Autodesk Inventor part; units mm, degrees
ref_plane "YZ Plane" through (0, 0, 0) normal (1, 0, 0) x (0, 1, 0)
ref_plane "XZ Plane" through (0, 0, 0) normal (0, 1, 0) x (-1, 0, 0)
ref_plane "XY Plane" through (0, 0, 0) normal (0, 0, 1) x (1, 0, 0)
sketch "スケッチ1" plane through (0, 0, 0) normal (0, 1, 0) x (-1, 0, 0)
  arc A0 (0, -155) -> (25, -152.9706) centre (0, 0) ccw
  line L0 (25, -152.9706) -> (0, 0)
  line L1 (0, 0) -> (0, -144.6885)
  arc A1 (9.5, -144.6885) -> (23.3871, -143.1015) centre (0, 0) ccw
  line L2 (9.5, -144.6885) -> (9.5, -122.5)
  line L3 (9.5, -122.5) -> (0, -122.5)
  arc A2 (-25, -152.9706) -> (0, -155) centre (0, 0) ccw
  line L4 (-25, -152.9706) -> (0, 0)
  arc A3 (-23.3871, -143.1015) -> (-9.5, -144.6885) centre (0, 0) ccw
  line L5 (-9.5, -144.6885) -> (-9.5, -122.5)
  line L6 (-9.5, -122.5) -> (0, -122.5)
  line L7 (9.5, -144.6885) -> (0, -144.6885) construction
  line L8 (-9.5, -144.6885) -> (0, -144.6885) construction
  line L9 (-9.5, -180.2611) -> (-9.5, 6.4286)
  line L10 (9.5, -180.2611) -> (9.5, 6.4286)
  line L11 (0, -130) -> (-3.1667, -130)
  line L12 (-3.1667, -130) -> (-3.1667, -125)
  line L13 (-3.1667, -125) -> (0, -125)
  line L14 (0, -130) -> (3.1667, -130)
  line L15 (3.1667, -130) -> (3.1667, -125)
  line L16 (3.1667, -125) -> (0, -125)
  line L17 (0, -144.6885) -> (0, -145)
  line L18 (0, -145) -> (0, -155)
  point P0 (0, -125)
  point P1 (0, -150)
  dimension "d4" = 19
  dimension "d12" = 122.5
  dimension "d13" = 10
  dimension "d29" = 19
  dimension "d32" = 5
  dimension "d33" = 6.3333
  dimension "d34" = 2.5
  dimension "d36" = 50
  dimension "d38" = 150
extrude "押し出し1" add sketch "スケッチ1" along normal blind 1.6 contours L18 L17 L1 L14 L15 L16 L3 L2 L10 A0 | A2 L9 L5 L6 L1 L13 L12 L11 L17 L18 | L10 A1 L0 A0 | A2 L4 A3 L9
sketch "スケッチ2" plane through (0, 1.6, 0) normal (0, 1, 0) x (1, 0, 0)
  line L0 (9.5, 122.5) -> (9.5, 144.6885)
  arc A0 (23.3871, 143.1015) -> (9.5, 144.6885) centre (0, 0) ccw
  line L1 (23.3871, 143.1015) -> (25, 152.9706)
  arc A1 (25, 152.9706) -> (-25, 152.9706) centre (0, 0) ccw
  line L2 (-25, 152.9706) -> (-23.3871, 143.1015)
  arc A2 (-9.5, 144.6885) -> (-23.3871, 143.1015) centre (0, 0) ccw
  line L3 (-9.5, 144.6885) -> (-9.5, 122.5)
  line L4 (-9.5, 122.5) -> (9.5, 122.5)
  line L5 (-9.5, 122.5) -> (5.5, 122.5)
  line L6 (5.5, 122.5) -> (5.5, 132.5)
  line L7 (5.5, 132.5) -> (-9.5, 132.5)
  line L8 (-9.5, 132.5) -> (-9.5, 122.5)
  line L9 (-6.3333, 127.5) -> (-3.1667, 127.5) construction
  line L10 (-6.3333, 127.5) -> (-9.5, 127.5) construction
  line L11 (-3.1667, 125) -> (-3.1667, 130)
  point P0 (6.3333, 127.5)
  dimension "d19" = 10
  dimension "d20" = 15
hole "穴1" at (6.3333, 1.6, -127.5) at (-6.3333, 1.6, -127.5) direction (0, -1, 0) diameter 2.4 depth 1.6
fillet "フィレット1" radius 10 2 edges at (9.5, 0.8, -144.6885) (-9.5, 0.8, -144.6885)
fillet "フィレット2" radius 1.5 4 edges at (-3.1667, 0.8, -130) (3.1667, 0.8, -125) (3.1667, 0.8, -130) (-3.1667, 0.8, -125)
properties part number "sensor" material "エポキシ樹脂"
Read the model definition and answer for the solid it produces. Units are mm, in the model's axes. A direction names the side the tool comes from. Give positions to 0.01 mm unless a question says otherwise; leave off trailing zeros. Loops run counter-clockwise (first coordinate to the right, second up) from the corner with the lowest first, then second, coordinate; pieces in that order, holes last. Notation, with made-up numbers: M 84,-25 L 111,-25 A16 ccw 111,-11 Z; hole C 18.25,62 d11. An arc over 180 degrees is marked long. Write each question's results on one line, items separated by ' | '.
1. Section C-C on y = 0.5 is taken. Give the vertices of the cut face in (x, z).
Values:
outline: M -25,-152.97 A155 ccw 0,-155 A155 ccw 25,-152.97 L 23.39,-143.1 A145.02 cw 20.94,-143.48 A10 cw 9.5,-133.58 L 9.5,-122.5 L -9.5,-122.5 L -9.5,-133.58 A10 cw -20.94,-143.48 A144.98 cw -23.39,-143.1 Z; hole C -6.33,-127.5 d2.4; hole M -3.17,-128.5 A1.5 ccw -1.67,-130 L 1.67,-130 A1.5 ccw 3.17,-128.5 L 3.17,-126.5 A1.5 ccw 1.67,-125 L -1.67,-125 A1.5 ccw -3.17,-126.5 Z; hole C 6.33,-127.5 d2.4
2. A tool of negligible diameter and unlimited length cuts with its end or side. For faces 1 (the face through (9.5, 1, -128)), 2 (the face through (0, 0, -142)), 3 (the face through (22.15, 0.79, -143.3)), 4 (the face through (2.74, 0.81, -129.55)), 5 (the face through (0, 1.6, -142)), from which of +Z, -Z, +X, -X, +Y, -Y can it reach the whole face along a straight path? Write none if from no direction.
Values:
face 1: +Z, +X, +Y, -Y | face 2: +Z, -Z, +X, -X, -Y | face 3: +Z, +Y, -Y | face 4: +Y, -Y | face 5: +Z, -Z, +X, -X, +Y
3. Section B-B on x = 7 is taken. Give the vertices of the cut face in (y, z), plus the area to 3 significant figures.
Values:
outline: M 0,-154.84 L 1.6,-154.84 L 1.6,-128.5 L 0,-128.5 Z; M 0,-126.5 L 1.6,-126.5 L 1.6,-122.5 L 0,-122.5 Z | area: 48.6 mm^2
4. The mould has two halves that part along Z. Classify faces 6 (the face through (-12.87, 0.81, -141.07)), 7 (the face through (-12.716, 0.789, -154.477)), 8 (the face through (-3.167, 1, -128)): pulls with the +Z half, pulls with the -Z half, needs draft (parallel to the pull), parting line crosses it, or undercut.
Values:
face 6: pulls with the +Z half | face 7: pulls with the -Z half | face 8: undercut
5. Straight lines are drawn through the part: line 1 (X direction, y = 0.8, z = -127.5); line 2 (Z direction, x = 0, y = 0.25); line 3 (X direction, y = 1.1, z = -131). For each, find the intervals that lie inside material, in ascending order. Write a range as [from, to].
Values:
line 1: x = [-9.5, -7.53], [-5.13, -3.17], [3.17, 5.13], [7.53, 9.5] | line 2: z = [-155, -130], [-125, -122.5] | line 3: x = [-9.5, 9.5]
6. Section D-D on z = -135.5 is taken. Give the vertices of the cut face in (x, y), plus the area to 3 significant figures.
Values:
outline: M -9.69,0 L 9.69,0 L 9.69,1.6 L -9.69,1.6 Z | area: 31.0 mm^2
7. Section A-A on z = -127.5 is taken. Give the vertices of the cut face in (x, y), plus the area to 3 significant figures.
Values:
outline: M -9.5,0 L -7.53,0 L -7.53,1.6 L -9.5,1.6 Z; M -5.13,0 L -3.17,0 L -3.17,1.6 L -5.13,1.6 Z; M 3.17,0 L 5.13,0 L 5.13,1.6 L 3.17,1.6 Z; M 7.53,0 L 9.5,0 L 9.5,1.6 L 7.53,1.6 Z | area: 12.6 mm^2
8. Given pin 1 (0.5 mm diameter, centred on y = 0.5, z = -127, fed in from -X); pin 2 (0.5 mm diameter, centred on y = 1, z = -125.5, fed in from +X); pin 3 (3 mm diameter, centred on x = 6.33, z = -127.5, fed in from +Y), each flat-ended and moving along its own axis, determine where each tip first touches the part or whether it passes through.
Values:
pin 1: stops at x = -9.5 | pin 2: stops at x = 9.5 | pin 3: stops at y = 1.6
